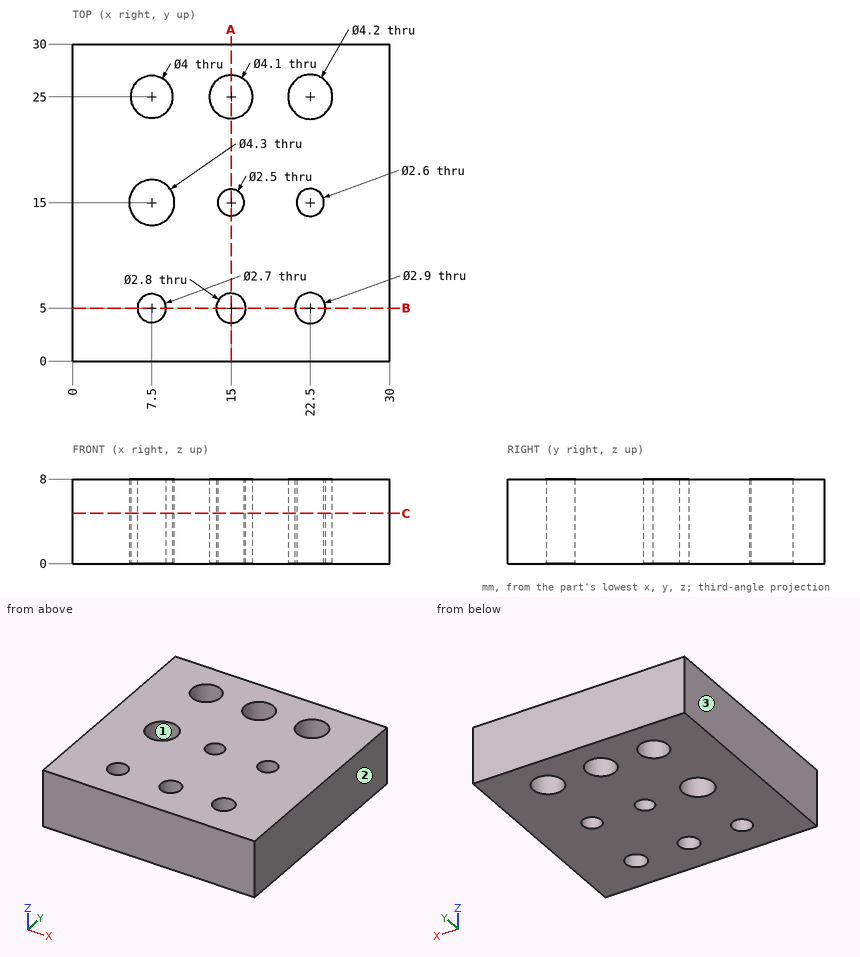
Here's the drawing with two shaded views (mm, measured from the low corner). I have some questions. Give positions to 0.01 mm unless a question says otherwise; leave off trailing zeros. Loops run counter-clockwise (first coordinate to the right, second up) from the corner with the lowest first, then second, coordinate; pieces in that order, holes last. Notation, with made-up numbers: M 68.25,89 L 73.25,89 A12 ccw 73.25,104 Z; hole C -1,-40 d1. An arc over 180 degrees is marked long. Answer in a Markdown table with one row per item.
1. Suppose I cut it at C-C on z = 4.75. Count the separate pieces of the cut face and the enclosed holes in it, plus the area to 3 significant figures.
Taken from the geometry:
| item | result |
|---|---|
| separate pieces | 1 |
| enclosed holes | 9 |
| area | 817 mm² |
2. Thinking about a two-plate mould opening in X: for the marked faces 1, 2 and 3, which applies, released by +X, released by -X, zero draft, split by the parting line, or undercut?
Taken from the geometry:
| item | result |
|---|---|
| face 1 | undercut |
| face 2 | released by +X |
| face 3 | released by -X |
3. Suppose I cut it at B-B on y = 5. Write out the boundary of the cut face in (x, z), plus the area to 3 significant figures.
Taken from the geometry:
| item | result |
|---|---|
| outline | M 0,0 L 6.15,0 L 6.15,8 L 0,8 Z; M 8.85,0 L 13.6,0 L 13.6,8 L 8.85,8 Z; M 16.4,0 L 21.05,0 L 21.05,8 L 16.4,8 Z; M 23.95,0 L 30,0 L 30,8 L 23.95,8 Z |
| area | 173 mm² |
4. If I drill on line 1 along Y through (x, z) = (22.5, 6); line 2 along Y through (x, z) = (7.5, 4); line 3 along X through (y, z) = (14, 7.25), over which ranges is the centre line in solid material (lowest first)?
Taken from the geometry:
| item | result |
|---|---|
| line 1 | y = 0 to 3.55, 6.45 to 13.7, 16.3 to 22.9, 27.1 to 30 |
| line 2 | y = 0 to 3.65, 6.35 to 12.85, 17.15 to 23, 27 to 30 |
| line 3 | x = 0 to 5.6, 9.4 to 14.25, 15.75 to 21.67, 23.33 to 30 |
5. Suppose I cut it at A-A on x = 15. Write out the boundary of the cut face in (y, z), plus the area to 3 significant figures.
Taken from the geometry:
| item | result |
|---|---|
| outline | M 0,0 L 3.6,0 L 3.6,8 L 0,8 Z; M 6.4,0 L 13.75,0 L 13.75,8 L 6.4,8 Z; M 16.25,0 L 22.95,0 L 22.95,8 L 16.25,8 Z; M 27.05,0 L 30,0 L 30,8 L 27.05,8 Z |
| area | 165 mm² |
